Design review of the part built by this model. Coordinates are the model's own, in mm. Give positions to 0.01 mm unless a question says otherwise; leave off trailing zeros. Order: outer loops, then holes, each group sorted by start corner. A loop starts at its lowest first (then second) coordinate and runs counter-clockwise, first axis right, second up. Notation, with made-up numbers: (49.5, -30.5) -> (72.5, -30.5) arc R24 cw to (72.5, -5.5) -> close; hole circle Ø4 at (-23, 69.25). An arc over 180 degrees is marked (long way). Return JSON: item names as keys, results as strings.
Autodesk Inventor part; units mm, degrees
ref_plane "YZ Plane" through (0, 0, 0) normal (1, 0, 0) x (0, 1, 0)
ref_plane "XZ Plane" through (0, 0, 0) normal (0, 1, 0) x (-1, 0, 0)
ref_plane "XY Plane" through (0, 0, 0) normal (0, 0, 1) x (1, 0, 0)
sketch "Sketch1" plane through (0, 0, 0) normal (0, 1, 0) x (-1, 0, 0)
  circle A0 centre (0, 0) radius 1.5
  dimension "d0" = 3
extrude "Extrusion1" add sketch "Sketch1" along normal blind 0.2
sketch "Sketch2" plane through (0, 0, 0) normal (0, 0, 1) x (1, 0, 0)
  line L0 (0, 0) -> (0, 0.1)
  line L1 (0, 0.1) -> (7, 0.1) construction
  line L2 (0, 0) -> (7, 0)
  line L3 (7, 0.2) -> (0, 0.2)
  arc A0 (0, 0.2) -> (0, 0) centre (0, 0.1) ccw
  arc A1 (7, 0) -> (7, 0.2) centre (7, 0.1) ccw
  line L4 (1.5, 0.2) -> (-1.5, 0.2)
  point P0 (3.5, 0.1)
  dimension "d3" = 0.1
  dimension "d4" = 7
  dimension "d5" = 0.2
extrude "Extrusion2" add sketch "Sketch2" along normal mid plane 3
pattern_circular "Circular Pattern1" count 6 over 360 about axis through (0, 0, 0) along (0, 1, 0) of "Extrusion2"
sketch "Sketch3" plane through (0, 0.2, 0) normal (0, 1, 0) x (1, 0, 0)
  circle A0 centre (0, 0) radius 0.5
  dimension "d11" = 1
extrude "Extrusion3" cut sketch "Sketch3" against normal blind 1
fillet "Fillet1" radius 2 6 edges at (0, 0.1, -3) (-2.5981, 0.1, -1.5) (-2.5981, 0.1, 1.5) (0, 0.1, 3) (2.5981, 0.1, 1.5) (2.5981, 0.1, -1.5)
properties part number "mid_7mm"
Item 1: Add section B-B (x = 0). Give the boundary of the cut face in (y, z).
Result set:
{"outline": "(0, -5) -> (0.2, -5) -> (0.2, -0.5) -> (0, -0.5) -> close; (0, 0.5) -> (0.2, 0.5) -> (0.2, 5) -> (0, 5) -> close"}
Item 2: Add section D-D (z = -4). Give the boundary of the cut face in (x, y).
Result set:
{"outline": "(-4.13, 0) -> (4.13, 0) -> (4.13, 0.2) -> (-4.13, 0.2) -> close"}
Item 3: Add section A-A (z = 0). Give the boundary of the cut face in (x, y), plus the area to 3 significant figures.
Result set:
{"outline": "(-7, 0) -> (-0.5, 0) -> (-0.5, 0.2) -> (-7, 0.2) arc R0.1 ccw to start; (0.5, 0) -> (7, 0) arc R0.1 ccw to (7, 0.2) -> (0.5, 0.2) -> close", "area": "2.63 mm^2"}
Item 4: Add section C-C (y = 0.1). Give the boundary of the cut face in (x, z).
Result set:
{"outline": "(-7.1, -1.5) -> (-6.06, -1.5) arc R2 cw to (-4.33, -4.5) -> (-4.85, -5.4) -> (-2.25, -6.9) -> (-1.73, -6) arc R2 cw to (1.73, -6) -> (2.25, -6.9) -> (4.85, -5.4) -> (4.33, -4.5) arc R2 cw to (6.06, -1.5) -> (7.1, -1.5) -> (7.1, 1.5) -> (6.06, 1.5) arc R2 cw to (4.33, 4.5) -> (4.85, 5.4) -> (2.25, 6.9) -> (1.73, 6) arc R2 cw to (-1.73, 6) -> (-2.25, 6.9) -> (-4.85, 5.4) -> (-4.33, 4.5) arc R2 cw to (-6.06, 1.5) -> (-7.1, 1.5) -> close; hole circle Ø1 at (0, 0)"}
Item 5: Wall thickness on L1, parallel to X at y = 0.1, z = 0; L2, parallel to Z at x = 0, y = 0.15; L3, parallel to X at y = 0.1, z = -5.5: over which ranges is each line inside the solid? List them lowest first. Write a range as [from, to].
Result set:
{"L1": "x = [-7.1, -0.5], [0.5, 7.1]", "L2": "z = [-5, -0.5], [0.5, 5]", "L3": "x = [-4.67, -1.32], [1.32, 4.67]"}
